```python
from build123d import *

# Parameters (mm, degrees)
SKETCH2_W           = 20.922356035
SKETCH2_H           = 22
BOSS_EXTRUDE1_DEPTH = 35
SKETCH3_R           = 1.5
CUT_EXTRUDE1_DEPTH  = 31
SKETCH7_W           = 2
SKETCH7_H           = 2.25
CUT_EXTRUDE3_DEPTH  = 22
SKETCH8_W           = 2
SKETCH8_H           = 2.25
CUT_EXTRUDE4_DEPTH  = 22
SKETCH11_R          = 1.5
SKETCH11_W          = 2.606017342
SKETCH11_H          = 18.048523845
SKETCH11_W_2        = 2.606017343
CUT_EXTRUDE5_DEPTH  = 36
FILLET2_R           = 1
BOSS_EXTRUDE2_REACH = 95.223
SKETCH12_W          = 2.606017343
SKETCH12_H          = 14.124057788
SKETCH12_W_2        = 2.606017342
CUT_EXTRUDE6_REACH  = 54.468
SKETCH13_W          = 3.309729442
SKETCH13_H          = 19.459110601
SKETCH13_W_2        = 3.249965826
SKETCH13_H_2        = 19.123541834


with BuildPart() as part:
    # Sketch2 → Boss-Extrude1 (new body)
    with BuildSketch(Plane(origin=(0, 0, 53.835350067), x_dir=(-1, 0, 0), z_dir=(0, 0, -1))):
        with Locations((9.484421134, 16.479237668)):
            Rectangle(SKETCH2_W, SKETCH2_H)
    extrude(amount=-BOSS_EXTRUDE1_DEPTH)

    # Sketch3 → Cut-Extrude1 (cut)
    with BuildSketch(Plane.ZY.offset(19.945599152)):
        with Locations((58.692130127, 16.479237668)):
            Circle(SKETCH3_R)
        with Locations((83.978570007, 16.479237668)):
            Circle(SKETCH3_R)
        with BuildLine():
            Line((62.585350067, 25.229237668), (62.585350067, 27.479237668))
            add(Edge.make_bspline(
                [(62.585350067, 5.479237668), (55.503237571, -7.59972181), (27.642884441, 16.75686213), (54.847177094, 35.965561503), (62.585350067, 27.479237668)],
                knots=[0, 0, 0, 0, 0.52323238, 1, 1, 1, 1], degree=3))
            Line((62.585350067, 5.479237668), (62.585350067, 7.729237668))
            ThreePointArc((62.585350067, 7.729237668), (56.398165732, 10.292053333), (53.835350067, 16.479237668))
            ThreePointArc((53.835350067, 16.479237668), (56.398165732, 22.666422004), (62.585350067, 25.229237668))
        make_face()
        with BuildLine():
            Line((80.085350067, 25.229237668), (80.085350067, 27.479237668))
            add(Edge.make_bspline(
                [(80.085350067, 5.479237668), (87.439945262, -7.310081119), (114.923859956, 16.481856124), (87.400752328, 40.475015582), (80.085350067, 27.479237668)],
                knots=[0, 0, 0, 0, 0.498892453, 1, 1, 1, 1], degree=3))
            Line((80.085350067, 5.479237668), (80.085350067, 7.729237668))
            ThreePointArc((80.085350067, 7.729237668), (86.272534402, 10.292053333), (88.835350067, 16.479237668))
            ThreePointArc((88.835350067, 16.479237668), (86.272534402, 22.666422004), (80.085350067, 25.229237668))
        make_face()
    extrude(amount=-CUT_EXTRUDE1_DEPTH, mode=Mode.SUBTRACT)

    # Sketch7 → Cut-Extrude3 (cut)
    with BuildSketch(Plane.ZY.offset(19.945599152)):
        with Locations((63.585350067, 26.354237668)):
            Rectangle(SKETCH7_W, SKETCH7_H)
        with Locations((79.085350067, 26.354237668)):
            Rectangle(SKETCH7_W, SKETCH7_H)
    extrude(amount=-CUT_EXTRUDE3_DEPTH, mode=Mode.SUBTRACT)

    # Sketch8 → Cut-Extrude4 (cut)
    with BuildSketch(Plane.ZY.offset(19.945599152)):
        with Locations((63.585350067, 6.604237668)):
            Rectangle(SKETCH8_W, SKETCH8_H)
        with Locations((79.085350067, 6.604237668)):
            Rectangle(SKETCH8_W, SKETCH8_H)
    extrude(amount=-CUT_EXTRUDE4_DEPTH, mode=Mode.SUBTRACT)

    # Sketch11 → Cut-Extrude5 (cut)
    with BuildSketch(Plane(origin=(0, 0, 53.835350067), x_dir=(-1, 0, 0), z_dir=(0, 0, -1))):
        with Locations(Location((9.484421134, 11.729237668, 0), (0, 0, 90))):
            Circle(SKETCH11_R)
        with Locations(Location((9.484421134, 21.23419775, 0), (0, 0, 90))):
            Circle(SKETCH11_R)
        with Locations((0.326251788, 16.479237669)):
            Rectangle(SKETCH11_W, SKETCH11_H)
        with Locations((18.642590481, 16.479237669)):
            Rectangle(SKETCH11_W_2, SKETCH11_H)
    extrude(amount=-CUT_EXTRUDE5_DEPTH, mode=Mode.SUBTRACT)

    # Fillet2
    fillet2_edges = [part.edges().sort_by_distance(p)[0] for p in [
        (-9.484421134, 27.479237668, 78.085350067),
    ]]
    fillet(fillet2_edges, radius=FILLET2_R)
    fillet2_2_edges = [part.edges().sort_by_distance(p)[0] for p in [
        (-9.484421134, 27.479237668, 64.585350067),
    ]]
    fillet(fillet2_2_edges, radius=FILLET2_R)
    fillet2_3_edges = [part.edges().sort_by_distance(p)[0] for p in [
        (-9.484421134, 7.729237668, 64.585350067),
    ]]
    fillet(fillet2_3_edges, radius=FILLET2_R)
    fillet2_4_edges = [part.edges().sort_by_distance(p)[0] for p in [
        (-9.484421134, 25.229237668, 64.585350067),
    ]]
    fillet(fillet2_4_edges, radius=FILLET2_R)
    fillet2_5_edges = [part.edges().sort_by_distance(p)[0] for p in [
        (-9.484421134, 25.229237668, 78.085350067),
    ]]
    fillet(fillet2_5_edges, radius=FILLET2_R)
    fillet2_6_edges = [part.edges().sort_by_distance(p)[0] for p in [
        (-9.484421134, 7.729237668, 78.085350067),
    ]]
    fillet(fillet2_6_edges, radius=FILLET2_R)
    fillet2_7_edges = [part.edges().sort_by_distance(p)[0] for p in [
        (-9.484421134, 5.479237668, 78.085350067),
    ]]
    fillet(fillet2_7_edges, radius=FILLET2_R)
    fillet2_8_edges = [part.edges().sort_by_distance(p)[0] for p in [
        (-9.484421134, 5.479237668, 64.585350067),
    ]]
    fillet(fillet2_8_edges, radius=FILLET2_R)

    # Boss-Extrude2: up to this face of the body (flat: up to its plane)
    boss_extrude2_end = Plane(part.part.faces().sort_by_distance((-18.642590481, 7.454975746, 71.335350067))[0])
    # Sketch12 → Boss-Extrude2 (add, up to the picked face)
    with BuildSketch(Plane.XZ.offset(-25.503499591), mode=Mode.PRIVATE) as boss_extrude2_sk1:
        with Locations((-18.642590481, 71.335350067)):
            Rectangle(SKETCH12_W, SKETCH12_H)
    boss_extrude2_tool1 = split(extrude(boss_extrude2_sk1.sketch, amount=BOSS_EXTRUDE2_REACH, mode=Mode.PRIVATE), bisect_by=boss_extrude2_end, keep=Keep.BOTH, mode=Mode.PRIVATE)
    # Sketch12 → Boss-Extrude2 (add, up to the picked face)
    with BuildSketch(Plane.XZ.offset(-25.503499591), mode=Mode.PRIVATE) as boss_extrude2_sk2:
        with Locations((-0.326251788, 71.335350067)):
            Rectangle(SKETCH12_W_2, SKETCH12_H)
    boss_extrude2_tool2 = split(extrude(boss_extrude2_sk2.sketch, amount=BOSS_EXTRUDE2_REACH, mode=Mode.PRIVATE), bisect_by=boss_extrude2_end, keep=Keep.BOTH, mode=Mode.PRIVATE)
    add(boss_extrude2_tool1.solids().sort_by(Axis((-18.64259, 25.5035, 71.33535), (0, -1, 0)))[0])
    add(boss_extrude2_tool2.solids().sort_by(Axis((-0.326252, 25.5035, 71.33535), (0, -1, 0)))[0])

    # Cut-Extrude6: up to this face of the body (flat: up to its plane)
    cut_extrude6_end = Plane(part.part.faces().sort_by_distance((-0.326251788, 16.479237668, 78.397378961))[0])
    # Sketch13 → Cut-Extrude6 (cut, up to the picked face)
    with BuildSketch(Plane(origin=(0, 0, 93.835350067), x_dir=(-1, 0, 0), z_dir=(0, 0, -1)), mode=Mode.PRIVATE) as cut_extrude6_sk1:
        with Locations((18.191565455, 16.712143076)):
            Rectangle(SKETCH13_W, SKETCH13_H)
    cut_extrude6_tool1 = split(extrude(cut_extrude6_sk1.sketch, amount=CUT_EXTRUDE6_REACH, mode=Mode.PRIVATE), bisect_by=cut_extrude6_end, keep=Keep.BOTH, mode=Mode.PRIVATE)
    # Sketch13 → Cut-Extrude6 (cut, up to the picked face)
    with BuildSketch(Plane(origin=(0, 0, 93.835350067), x_dir=(-1, 0, 0), z_dir=(0, 0, -1)), mode=Mode.PRIVATE) as cut_extrude6_sk2:
        with Locations((1.015942541, 16.59296095)):
            Rectangle(SKETCH13_W_2, SKETCH13_H_2)
    cut_extrude6_tool2 = split(extrude(cut_extrude6_sk2.sketch, amount=CUT_EXTRUDE6_REACH, mode=Mode.PRIVATE), bisect_by=cut_extrude6_end, keep=Keep.BOTH, mode=Mode.PRIVATE)
    add(cut_extrude6_tool1.solids().sort_by(Axis((-18.191565, 16.712143, 93.83535), (0, 0, -1)))[0], mode=Mode.SUBTRACT)
    add(cut_extrude6_tool2.solids().sort_by(Axis((-1.015943, 16.592961, 93.83535), (0, 0, -1)))[0], mode=Mode.SUBTRACT)


solid = part.part
```
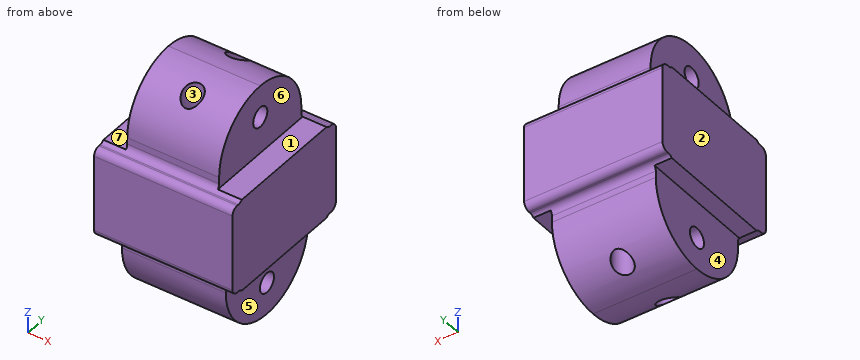
Here's how the part is built. I have some questions about the finished solid (model axes, mm). Face numbers are marked on the shaded views. A direction names the side the tool comes from. Give positions to 0.01 mm unless a question says otherwise; leave off trailing zeros. Order: outer loops, then holes, each group sorted by start corner. A loop starts at its lowest first (then second) coordinate and runs counter-clockwise, first axis right, second up. Notation, with made-up numbers: (12.5, -35) - (41.5, -35) arc R21 ccw to (41.5, -29) - close; hole circle Ø11 at (-23.5, 77.5). An arc over 180 degrees is marked (long way). Answer as a JSON object with one key per item and string values. Group by question number.
Item 1: If we section it at C-C on x = -0.25: Please give me the cut outline in (y, z).
Item 2: If we section it at B-B on x = -12.75: Please give me the cut outline in (y, z).
Item 3: If we mould it in two halves opening along X, with no side actions, what happens to the marked faces 1, 2 and 3? For each: pulls with the +X half, pulls with the -X half, needs draft (parallel to the pull), parting line crosses it, or undercut.
Item 4: For P1, Ø10, axis at x = -9, y = 23, coming from the -Z side; P2, Ø11.5, axis at y = 17, z = 85, coming from the +X side; P3, Ø2, axis at x = -3.5, y = 23.5, coming from the +Z side, each with a flat end and sliding along its axis, tell me the tip position at first contact or that it passes through.
Item 5: Please list where these lines run through material, in increasing order: probe 1 along Z at (x, y) = (-7.25, 17.25); probe 2 along X at (y, z) = (17, 79.5); probe 3 along Z at (x, y) = (-10.5, 17.75).
Item 6: If we section it at A-A on z = 85: Please give me the cut outline in (x, y), and give its area (3 significant figures).
Item 7: If we section it at D-D on y = 20.5: Please give me the cut outline in (x, z), and give its area (3 significant figures).
Item 8: Which directions (+Z, -Z, +X, -X, +Y, -Y) give clear straight access to the entire face, cutting with the end or side of a thin tool? Please do the marked faces 4, 5, 6 and 7.
Result set:
{
 "1": {"outline": "(5.48, 65.59) arc R1 ccw to (6.48, 64.59) - (6.73, 64.59) arc R1 cw to (7.45, 64.27) - (25.5, 64.27) arc R1 cw to (26.23, 64.59) - (26.48, 64.59) arc R1 ccw to (27.48, 65.59) - (27.48, 77.09) arc R1 ccw to (26.48, 78.09) - (26.23, 78.09) arc R1 cw to (25.5, 78.4) - (7.45, 78.4) arc R1 cw to (6.73, 78.09) - (6.48, 78.09) arc R1 ccw to (5.48, 77.09) - close"},
 "2": {"outline": "(5.48, 65.59) arc R1 ccw to (6.48, 64.59) - (6.73, 64.59) arc R1 cw to (7.73, 63.59) - (7.73, 62.59) arc R8.75 ccw to (25.23, 62.59) - (25.23, 63.59) arc R1 cw to (26.23, 64.59) - (26.48, 64.59) arc R1 ccw to (27.48, 65.59) - (27.48, 77.09) arc R1 ccw to (26.48, 78.09) - (26.23, 78.09) arc R1 cw to (25.23, 79.09) - (25.23, 80.09) arc R8.75 ccw to (7.73, 80.09) - (7.73, 79.09) arc R1 cw to (6.73, 78.09) - (6.48, 78.09) arc R1 ccw to (5.48, 77.09) - close; hole circle Ø3 at (16.48, 58.69); hole circle Ø3 at (16.48, 83.98)"},
 "3": {"face 1": "needs draft", "face 2": "pulls with the -X half", "face 3": "undercut"},
 "4": {"P1": "z = 53.97", "P2": "x = -2.64", "P3": "z = 86.43"},
 "5": {"probe 1": "53.87 to 57.41, 59.98 to 82.69, 85.27 to 88.8", "probe 2": "-16.54 to -2.64", "probe 3": "53.93 to 57.9, 59.49 to 83.18, 84.78 to 88.74"},
 "6": {"outline": "(-16.54, 9.24) - (-2.64, 9.24) - (-2.64, 15.38) - (-16.54, 15.38) - close; (-16.54, 17.58) - (-2.64, 17.58) - (-2.64, 23.72) - (-16.54, 23.72) - close; hole circle Ø3 at (-9.48, 11.73); hole circle Ø3 at (-9.48, 21.23)", "area": "157 mm²"},
 "7": {"outline": "(-19.95, 64.27) - (-17.34, 64.27) - (-17.34, 54.81) - (-10.79, 54.81) - (-10.79, 87.86) - (-16.54, 87.86) - (-16.54, 78.4) - (-19.95, 78.4) - close; (-8.18, 54.81) - (-1.63, 54.81) - (-1.63, 64.27) - (0.98, 64.27) - (0.98, 78.4) - (-2.64, 78.4) - (-2.64, 87.86) - (-8.18, 87.86) - close", "area": "489 mm²"},
 "8": {"face 4": "-Z, -X, +Y, -Y", "face 5": "-Z, +X, +Y, -Y", "face 6": "+Z, +X, +Y, -Y", "face 7": "+Z, -X, +Y, -Y"}
}
